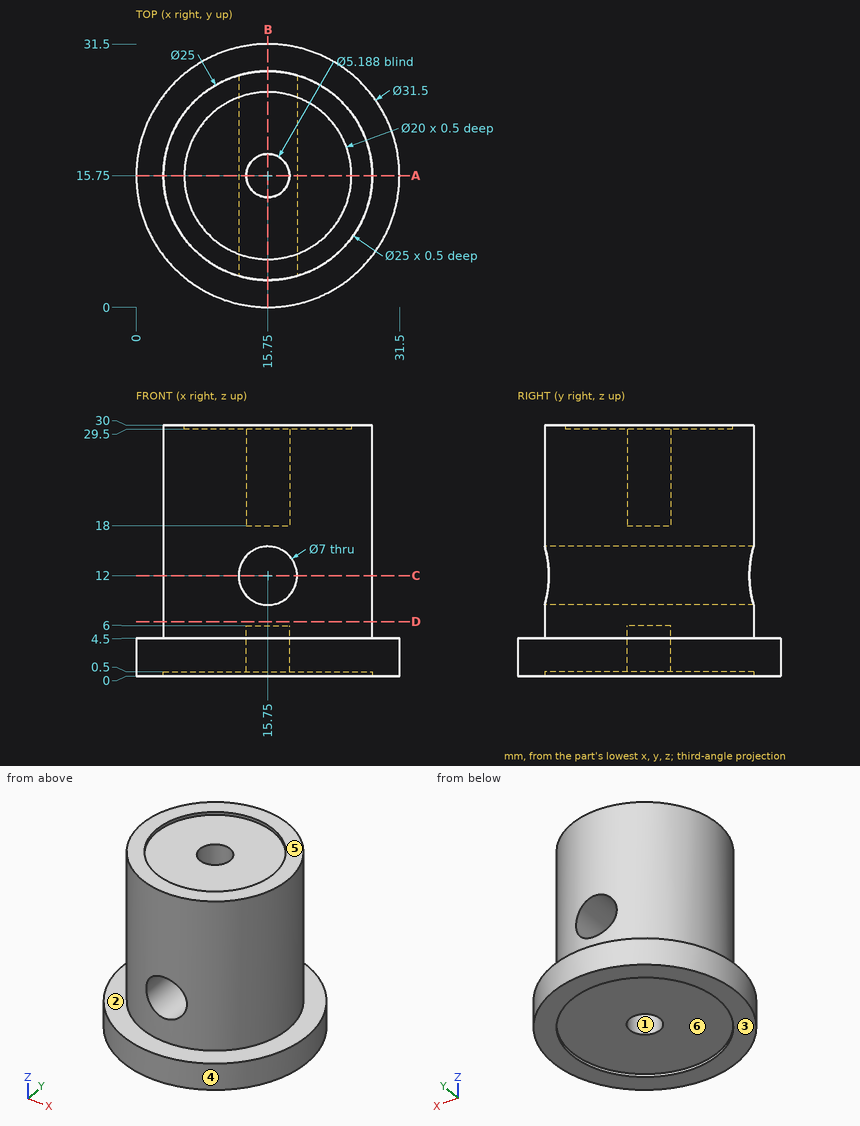
Print and shaded views of the part. All mm, measured from the part's lowest x, y and z. A direction names the side the tool comes from. Coordinates: 2 decimals unless noted, no trailing zeros. Loops run counter-clockwise (first coordinate to the right, second up) from the corner with the lowest first, then second, coordinate; pieces in that order, holes last. Notation, with made-up numbers: M 7,-20.5 L 34,-20.5 A19 cw 34,13.5 Z; hole C 25,-10 d9. An arc over 180 degrees is marked long. Use a Markdown table: item, result. Add a question column.
Q1. Cut at A-A (y = 15.75). Write the cut outline in (x, z).
Q2. Which spindle directions (+Z, -Z, +X, -X, +Y, -Y) get a long thin tool onto all of the face, cutting with end or side? Do the marked faces 1, 2 and 3. Say none if no direction does.
Q3. Cut at D-D (z = 6.5). Write the cut outline in (x, y).
Q4. Pin check, flat tips, straight feed: P1, Ø11, axis at x = 15.75, z = 12, coming from the -Y side; P2, Ø7.5, axis at x = 18.5, y = 15, coming from the -Z side; P3, Ø1, axis at x = 15.5, z = 7, coming from the +Y side. Stop position of each tip, or through.
Q5. Cut at C-C (z = 12). Write the cut outline in (x, y), and give its area (3 significant figures).
Q6. Probe L1, parallel to Z at x = 16, y = 27; L2, parallel to Z at x = 15.5, y = 11; L3, parallel to Y at x = 15.75, z = 0.3. List the from-to ranges inside material, lowest first.
Q7. Cut at B-B (x = 15.75). Write the cut outline in (y, z), and give its area (3 significant figures).
Q8. Mould opens along X. For the marked faces 4, 5 and 6 say: +X half, -X half, draft (parallel to the pull), parting line (faces both ways), or undercut.
Worked out:
| question | item | result |
|---|---|---|
| 1 | outline | M 0,0 L 3.25,0 L 3.25,0.5 L 13.16,0.5 L 13.16,6 L 18.34,6 L 18.34,0.5 L 28.25,0.5 L 28.25,0 L 31.5,0 L 31.5,4.5 L 28.25,4.5 L 28.25,30 L 25.75,30 L 25.75,29.5 L 18.34,29.5 L 18.34,18 L 13.16,18 L 13.16,29.5 L 5.75,29.5 L 5.75,30 L 3.25,30 L 3.25,4.5 L 0,4.5 Z; hole C 15.75,12 d7 |
| 2 | face 1 | -Z |
| 2 | face 2 | +Z |
| 2 | face 3 | -Z, +X, -X, +Y, -Y |
| 3 | outline | C 15.75,15.75 d25 |
| 4 | P1 | stops at y = 3.25 |
| 4 | P2 | stops at z = 0.5 |
| 4 | P3 | stops at y = 28.25 |
| 5 | outline | M 12.25,3.75 L 12.25,27.75 A12.5 ccw Z; M 19.25,3.75 A12.5 ccw 19.25,27.75 Z |
| 5 | area | 318 mm2 |
| 6 | L1 | z = 0.5 to 8.51, 15.49 to 30 |
| 6 | L2 | z = 0.5 to 8.51, 15.49 to 29.5 |
| 6 | L3 | y = 0 to 3.25, 28.25 to 31.5 |
| 7 | outline | M 0,0 L 3.25,0 L 3.25,0.5 L 13.16,0.5 L 13.16,6 L 18.34,6 L 18.34,0.5 L 28.25,0.5 L 28.25,0 L 31.5,0 L 31.5,4.5 L 28.25,4.5 L 28.25,8.5 L 3.25,8.5 L 3.25,4.5 L 0,4.5 Z; M 3.25,15.5 L 28.25,15.5 L 28.25,30 L 25.75,30 L 25.75,29.5 L 18.34,29.5 L 18.34,18 L 13.16,18 L 13.16,29.5 L 5.75,29.5 L 5.75,30 L 3.25,30 Z |
| 7 | area | 494 mm2 |
| 8 | face 4 | parting line |
| 8 | face 5 | draft |
| 8 | face 6 | undercut |
